```python
from build123d import *

# Parameters (mm, degrees)
F0_R     = 9.525
F1_DEPTH = 2.54
F3_DEPTH = 1.905


with BuildPart() as f1:
    # F0 (on Top) → F1 (new body)
    with BuildSketch(Plane.XY):
        Circle(F0_R)
    extrude(amount=F1_DEPTH)

    # F2 (on Top) → F3 (cut)
    with BuildSketch(Plane.XY):
        Polygon((1.143, 4.699), (-1.143, 4.699), (-1.143, 1.143), (-4.699, 1.143), (-4.699, -1.143), (-1.143, -1.143), (-1.143, -4.699), (1.143, -4.699), (1.143, -1.143), (4.699, -1.143), (4.699, 1.143), (1.143, 1.143), align=None)
    extrude(amount=F3_DEPTH, mode=Mode.SUBTRACT)


solid = f1.part
```
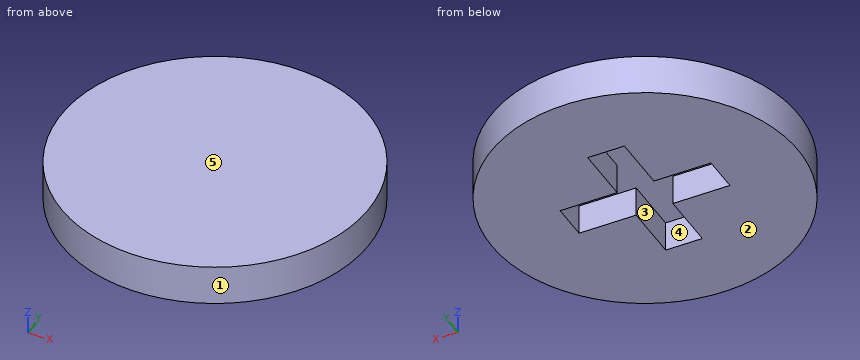
The model under review builds one solid part; all positions refer to its coordinate system, in mm. Face numbers are marked on the shaded views. A direction names the side the tool comes from. Give positions to 0.01 mm unless a question says otherwise; leave off trailing zeros. Write each loop counter-clockwise with the first axis right and the second up, starting at its lowest first coordinate (ties: lowest second). Pieces come first, ordered by that corner, then holes. Notation, with made-up numbers: (0.5, -5) - (43.5, -5) arc R16 ccw to (43.5, 17) - close; hole circle Ø3 at (-0.5, 12.25). An arc over 180 degrees is marked (long way). Answer in a Markdown table with one row per item. Add a question column.
1. We need section A-A on x = 0. Write out the cut boundary in (y, z) (3 decimals).
2. We need section B-B on z = 1.45. Write out the cut boundary in (x, y) (3 decimals), then the cut area to 3 significant figures.
3. Tool access review of the marked faces 4 and 5: name each direction out of +Z, -Z, +X, -X, +Y, -Y from which nothing blocks a thin tool from reaching the whole face with its end or side.
4. Insertion check: P1, Ø1.5, axis at x = 7.5, z = 1, coming from the -Y side; P2, Ø1.5, axis at x = 2.5, z = 0.5, coming from the -Y side; P3, Ø1, axis at x = -2.5, z = 1.5, coming from the -Y side. Each pin has a flat end and moves straight along its axis. Give the tip position at first contact, or say it passes through.
5. We need section D-D on x = 8. Write out the cut boundary in (y, z), then the cut area to 3 significant figures.
6. Draft analysis for pull direction Y (two halves, no side actions). For the marked faces 1, 2 and 3, state which applies: +Y half, -Y half, draft (parallel to the pull), parting line (faces both ways), or undercut.
7. Wall thickness on line 1 along Z through (x, y) = (4.5, -0.5) (3 decimals); line 2 along X through (y, z) = (3.5, 1.15); line 3 along X through (y, z) = (1.5, 1.4): over which ranges is each line inside the solid? List them lowest first. Write a range as [from, to].
Ans:
| question | item | result |
|---|---|---|
| 1 | outline | (-9.525, 0) - (-4.699, 0) - (-4.699, 1.905) - (4.699, 1.905) - (4.699, 0) - (9.525, 0) - (9.525, 2.54) - (-9.525, 2.54) - close |
| 2 | outline | circle Ø19.05 at (0, 0); hole (-4.699, -1.143) - (-1.143, -1.143) - (-1.143, -4.699) - (1.143, -4.699) - (1.143, -1.143) - (4.699, -1.143) - (4.699, 1.143) - (1.143, 1.143) - (1.143, 4.699) - (-1.143, 4.699) - (-1.143, 1.143) - (-4.699, 1.143) - close |
| 2 | area | 247 mm^2 |
| 3 | face 4 | -Z |
| 3 | face 5 | +Z, +X, -X, +Y, -Y |
| 4 | P1 | stops at y = -6.72 |
| 4 | P2 | stops at y = -9.36 |
| 4 | P3 | stops at y = -9.31 |
| 5 | outline | (-5.17, 0) - (5.17, 0) - (5.17, 2.54) - (-5.17, 2.54) - close |
| 5 | area | 26.3 mm^2 |
| 6 | face 1 | parting line |
| 6 | face 2 | draft |
| 6 | face 3 | undercut |
| 7 | line 1 | z = [1.905, 2.54] |
| 7 | line 2 | x = [-8.86, -1.14], [1.14, 8.86] |
| 7 | line 3 | x = [-9.41, -1.14], [1.14, 9.41] |
